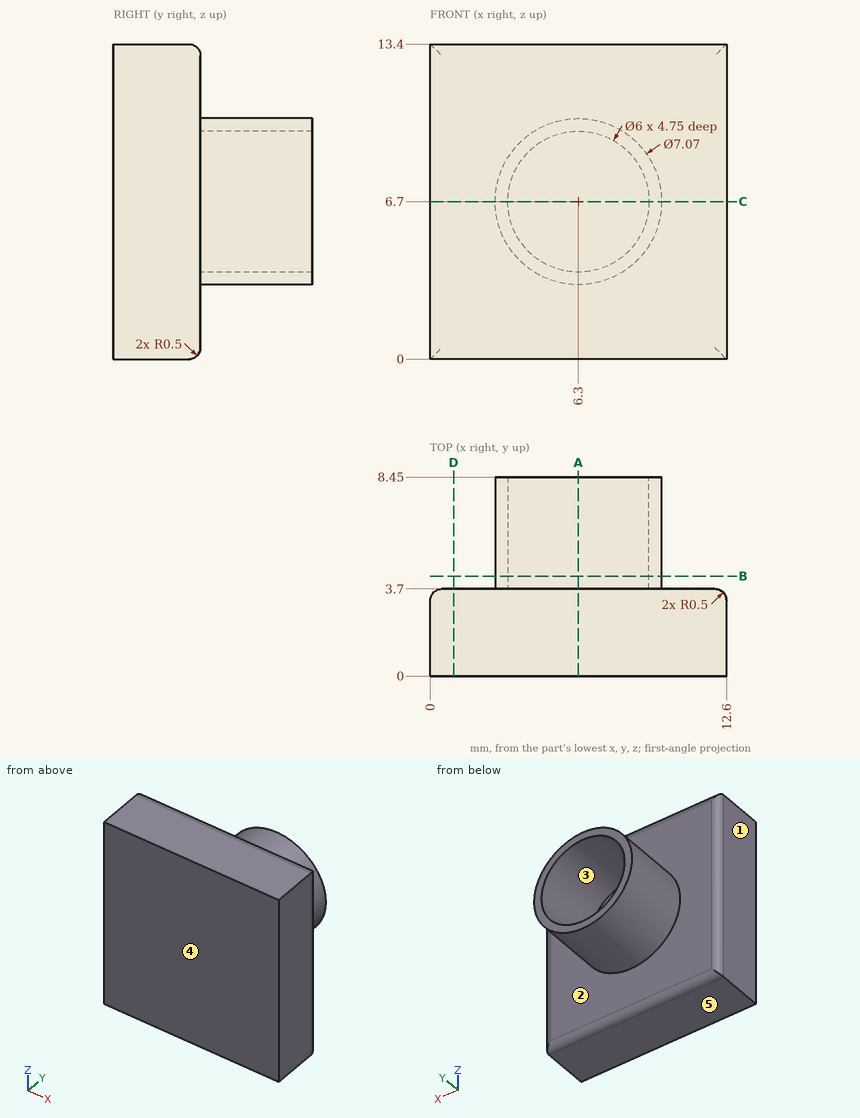
Answer from the drawing. Dimensions are ordinates in mm from the lowest x, y and z of the part. A direction names the side the tool comes from. Coordinates: 2 decimals unless noted, no trailing zeros. Loops run counter-clockwise (first coordinate to the right, second up) from the corner with the lowest first, then second, coordinate; pieces in that order, holes last.
Q1. Each of these flat-tipped pins is pushed along its axis until it touches: pin 1 Ø2 at (y, z) = (6, 6.5) entering from -X (3 decimals); pin 2 Ø1.5 at (y, z) = (4, 4) entering from -X; pin 3 Ø4 at (x, y) = (8.5, 7) entering from -Z. Where does it stop, or does it pass through?
Q2. The mould has two halves that part along Z. Classify the marked faces 3, 4 and 5: +Z half, -Z half, draft (parallel to the pull), parting line (faces both ways), or undercut.
Q3. The part is cut by section A-A on x = 6.3. Write down the section's boundary in (y, z) (3 decimals), and give its area (3 significant figures).
Q4. The part is cut by section C-C on z = 6.7. Write down the section's boundary in (x, y) (3 decimals), and give its area (3 significant figures).
Q5. Consider probe 1 along Z at (x, y) = (6.3, 7) (3 decimals); probe 2 along Y at (x, z) = (4.25, 11.25); probe 3 along X at (y, z) = (8.25, 4.5). Determine where each line is inside the solid, lowest interval first.
Q6. The part is cut by section B-B on y = 4.25. Write down the section's boundary in (x, z) (3 decimals).
Q7. The part is cut by section D-D on x = 1. Write down the section's boundary in (y, z), and give its area (3 significant figures).
Q8. Which of the six approach directions +Z, -Z, +X, -X, +Y, -Y give full straight-line access (tool end or side, diameter ignored) to the marked faces 1 and 2?
Results below:
1. pin 1: stops at x = 2.765
1. pin 2: stops at x = 0
1. pin 3: stops at z = 3.17
2. face 3: undercut
2. face 4: draft
2. face 5: -Z half
3. outline: (0, 0) - (3.2, 0) arc R0.5 ccw to (3.7, 0.5) - (3.7, 3.165) - (8.45, 3.165) - (8.45, 3.7) - (3.7, 3.7) - (3.7, 9.7) - (8.45, 9.7) - (8.45, 10.235) - (3.7, 10.235) - (3.7, 12.9) arc R0.5 ccw to (3.2, 13.4) - (0, 13.4) - close
3. area: 54.6 mm2
4. outline: (0, 0) - (12.6, 0) - (12.6, 3.2) arc R0.5 ccw to (12.1, 3.7) - (9.835, 3.7) - (9.835, 8.45) - (9.3, 8.45) - (9.3, 3.7) - (3.3, 3.7) - (3.3, 8.45) - (2.765, 8.45) - (2.765, 3.7) - (0.5, 3.7) arc R0.5 ccw to (0, 3.2) - close
4. area: 51.6 mm2
5. probe 1: z = 3.165 to 3.7, 9.7 to 10.235
5. probe 2: y = 0 to 3.7
5. probe 3: x = 3.53 to 4.26, 8.34 to 9.07
6. outline: circle Ø7.07 at (6.3, 6.7); hole circle Ø6 at (6.3, 6.7)
7. outline: (0, 0) - (3.2, 0) arc R0.5 ccw to (3.7, 0.5) - (3.7, 12.9) arc R0.5 ccw to (3.2, 13.4) - (0, 13.4) - close
7. area: 49.5 mm2
8. face 1: +Z, -Z, -X, +Y, -Y
8. face 2: +Y
